from build123d import *

# Parameters (mm, degrees)
SKETCH1_W                       = 400
SKETCH1_H                       = 200
BASE_FLANGE1_DEPTH              = 10
BREAK_CORNER1_DEPTH             = 10
M10_CLEARANCE_HOLE1_D           = 12
M10_CLEARANCE_HOLE1_CSINK_D     = 12.05
M10_CLEARANCE_HOLE1_CSINK_ANGLE = 90
FILLET1_R                       = 3


# Read off the part's stored shape, not the designer's step: Break-Corner1
# Sheet-metal steps are written as plain solids
with BuildPart() as part:
    # Sketch1 → Base-Flange1 (new body)
    with BuildSketch(Plane(origin=(0, 0, 0), x_dir=(1, 0, 0), z_dir=(0, 1, 0))):
        Rectangle(SKETCH1_W, SKETCH1_H)
    extrude(amount=BASE_FLANGE1_DEPTH)

    # Break-Corner1 outline → Break-Corner1 (cut)
    with BuildSketch(Plane(origin=(0, 0, 0), x_dir=(1, 0, 0), z_dir=(0, 1, 0))):
        Polygon((200, -100), (200, -90), (190, -100), align=None)
        Polygon((190, 100), (200, 90), (200, 100), align=None)
    extrude(amount=BREAK_CORNER1_DEPTH, mode=Mode.SUBTRACT)

    # M10 Clearance Hole1 (through all)
    with Locations(Plane(origin=(0, 10, 0), x_dir=(1, 0, 0), z_dir=(0, 1, 0))):
        with Locations((-50, 40), (10, 40), (70, 40), (130, 40), (130, 0), (130, -40), (70, -40), (10, -40), (-50, -40)):
            CounterSinkHole(M10_CLEARANCE_HOLE1_D / 2, M10_CLEARANCE_HOLE1_CSINK_D / 2, counter_sink_angle=M10_CLEARANCE_HOLE1_CSINK_ANGLE)

    # Fillet1
    fillet1_edges = [part.edges().sort_by_distance(p)[0] for p in [
        (200, 0, 0),
        (200, 10, 0),
        (200, 5, 90),
        (195, 0, 95),
        (190, 5, 100),
        (195, 10, 95),
        (-5, 0, -100),
        (-5, 10, -100),
        (190, 5, -100),
        (195, 0, -95),
        (200, 5, -90),
        (195, 10, -95),
        (-5, 0, 100),
        (-200, 5, -100),
        (-200, 5, 100),
        (-5, 10, 100),
    ]]
    fillet(fillet1_edges, radius=FILLET1_R)


solid = part.part
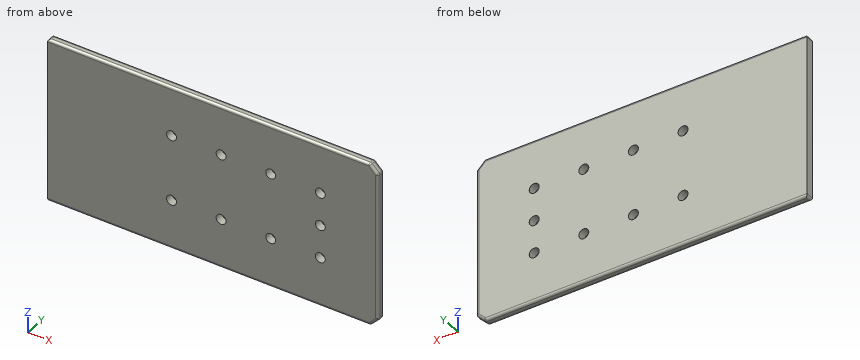
Check sheet for the modelled part. Datum: model origin and axes. Units: mm. Give positions to 0.01 mm unless a question says otherwise; leave off trailing zeros. Write each loop counter-clockwise with the first axis right and the second up, starting at its lowest first coordinate (ties: lowest second). Pieces come first, ordered by that corner, then holes. Notation, with made-up numbers: (-29.75, 75.25) -> (-20.75, 75.25) arc R24 cw to (-20.75, 105.25) -> close; hole circle Ø6 at (67, 84). An arc over 180 degrees is marked (long way). Write item = value, one per line.
Item 1: Gauge pin test, flat ends, axial feed: pin 1 (7 mm diameter, centred on x = 130, z = 40, fed in from +Y); pin 2 (3 mm diameter, centred on x = 105, y = 9, fed in from -Z). Record the tip position at first contact, or that the pin passes through.
Output:
pin_1 = through
pin_2 = -99.96
Item 2: Sectioned sample at A-A on x = 130. Record the boundary of the cut face in (y, z) (3 decimals).
Output:
outline = (0, -97) arc R3 ccw to (3, -100) -> (7, -100) arc R3 ccw to (10, -97) -> (10, -46.025) -> (9.975, -46) -> (0, -46) -> close; (0, -34) -> (9.975, -34) -> (10, -33.975) -> (10, -6.025) -> (9.975, -6) -> (0, -6) -> close; (0, 6) -> (9.975, 6) -> (10, 6.025) -> (10, 33.975) -> (9.975, 34) -> (0, 34) -> close; (0, 46) -> (9.975, 46) -> (10, 46.025) -> (10, 97) arc R3 ccw to (7, 100) -> (3, 100) arc R3 ccw to (0, 97) -> close
Item 3: Sectioned sample at C-C on x = 70. Record the boundary of the cut face in (y, z) (3 decimals), and give its area (3 significant figures).
Output:
outline = (0, -97) arc R3 ccw to (3, -100) -> (7, -100) arc R3 ccw to (10, -97) -> (10, -46.025) -> (9.975, -46) -> (0, -46) -> close; (0, -34) -> (9.975, -34) -> (10, -33.975) -> (10, 33.975) -> (9.975, 34) -> (0, 34) -> close; (0, 46) -> (9.975, 46) -> (10, 46.025) -> (10, 97) arc R3 ccw to (7, 100) -> (3, 100) arc R3 ccw to (0, 97) -> close
area = 1,750 mm^2
Item 4: Scan lines: probe 1 along Z at (x, y) = (10, 6.5); probe 2 along X at (y, z) = (7.25, -40); probe 3 along Z at (x, y) = (65, 1.75). Record each from-to range of solid material in increasing order. Write a range as from..to.
Output:
probe_1 = -100..-46, -34..34, 46..100
probe_2 = -200..-56, -44..4, 16..64, 76..124, 136..199.99
probe_3 = -99.73..-43.32, -36.68..36.68, 43.32..99.73
Item 5: Sectioned sample at B-B on z = 40. Count the separate pieces of the cut face and the enclosed holes in it, and give its area (3 significant figures).
Output:
separate_pieces = 5
enclosed_holes = 0
area = 3,520 mm^2
